Model file for the job. Use its own axes, mm. A direction names the side the tool comes from. Coordinates: 2 decimals unless noted, no trailing zeros. Write each loop counter-clockwise with the first axis right and the second up, starting at its lowest first coordinate (ties: lowest second). Pieces come first, ordered by that corner, then holes. Notation, with made-up numbers: M 28.25,75 L 80.25,75 A32 ccw 80.25,113 Z; hole C 29.25,84.5 d6. An arc over 180 degrees is marked long. Put each result on its own line as item: value. Start each with the question number.
Q1. Drop flat-ended pins along their axis: pin 1 (2.5 mm diameter, centred on x = 0.5, z = 25.5, fed in from +Y); pin 2 (1 mm diameter, centred on y = 1, z = 28.5, fed in from -X); pin 3 (1.5 mm diameter, centred on x = -1.5, z = 19.5, fed in from +Y). Give the stop position or say it passes through.
Q2. Cut at B-B (z = 13.5). Write the cut outline in (x, y).
Q3. Which spindle directions (+Z, -Z, +X, -X, +Y, -Y) get a long thin tool onto all of the face, cutting with end or side? Do faces 4 (the flat face through (0, 2, 8)), 5 (the cylindrical face through (-2.8, 0.1, 34.6)), 6 (the cylindrical face through (-3, 0.1, 35.2)). Say none if no direction does.
Q4. Pull direction Z, two halves, no side cores. Call faces 1 (the cylindrical face through (-0.65, -2.93, 17.77)), 2 (the flat face through (0, 1.5, 10)), 3 (the flat face through (0, 0, 36)): pulls with the +Z half, pulls with the -Z half, needs draft (parallel to the pull), parting line crosses it, or undercut.
Q5. Drill centre lines: line 1 along Z through (x, y) = (-1.7, 1.65); line 2 along X through (y, z) = (0.15, 4); line 3 along Y through (x, z) = (2.2, 2.5). Where is each one in solid material? Low to high.
Q6. Cut at C-C (y = 2). Give the number of separate pieces and of enclosed holes in the cut face, then the cut area to 3 significant figures.
```python
from build123d import *

# Parameters (mm, degrees)
SZKIC1_R                    = 3
DODANIE_WYCI_GNI_CIE1_DEPTH = 36
SFAZOWANIE1_SIZE            = 0.5
WYTNIJ_WYCI_GNI_CIE1_START  = -1.7
SZKIC2_R                    = 3
SZKIC2_R_2                  = 2.8
WYTNIJ_WYCI_GNI_CIE1_DEPTH  = 0.7
WYTNIJ_WYCI_GNI_CIE2_START  = -1
SZKIC3_R                    = 3
SZKIC3_R_2                  = 2.8
WYTNIJ_WYCI_GNI_CIE2_DEPTH  = 0.7
WYTNIJ_WYCI_GNI_CIE3_START  = -13
WYTNIJ_WYCI_GNI_CIE3_DEPTH  = 5
WYTNIJ_WYCI_GNI_CIE4_START  = -28
WYTNIJ_WYCI_GNI_CIE4_DEPTH  = 5


with BuildPart() as part:
    # Szkic1 → Dodanie-wyci_gni_cie1 (new body)
    with BuildSketch(Plane.XY):
        Circle(SZKIC1_R)
    extrude(amount=DODANIE_WYCI_GNI_CIE1_DEPTH)

    # Sfazowanie1
    sfazowanie1_edges = [part.edges().sort_by_distance(p)[0] for p in [
        (-3, 0, 0),
        (-3, 0, 36),
    ]]
    chamfer(sfazowanie1_edges, length=SFAZOWANIE1_SIZE)

    # Szkic2 → Wytnij-wyci_gni_cie1 (cut)
    with BuildSketch(Plane.XY.offset(36).offset(WYTNIJ_WYCI_GNI_CIE1_START)):
        Circle(SZKIC2_R)
        Circle(SZKIC2_R_2, mode=Mode.SUBTRACT)
    extrude(amount=WYTNIJ_WYCI_GNI_CIE1_DEPTH, mode=Mode.SUBTRACT)

    # Szkic3 → Wytnij-wyci_gni_cie2 (cut)
    with BuildSketch(Plane(origin=(0, 0, 0), x_dir=(-1, 0, 0), z_dir=(0, 0, -1)).offset(WYTNIJ_WYCI_GNI_CIE2_START)):
        Circle(SZKIC3_R)
        with Locations(Location((0, 0, 0), (0, 0, 180))):
            Circle(SZKIC3_R_2, mode=Mode.SUBTRACT)
    extrude(amount=-WYTNIJ_WYCI_GNI_CIE2_DEPTH, mode=Mode.SUBTRACT)

    # Szkic4 → Wytnij-wyci_gni_cie3 (cut)
    with BuildSketch(Plane.XY.offset(36).offset(WYTNIJ_WYCI_GNI_CIE3_START)):
        with BuildLine():
            Line((-2.598076211, 1.5), (2.598076211, 1.5))
            ThreePointArc((2.598076211, 1.5), (0, 3), (-2.598076211, 1.5))
        make_face()
    extrude(amount=WYTNIJ_WYCI_GNI_CIE3_DEPTH, mode=Mode.SUBTRACT)

    # Szkic4_2 → Wytnij-wyci_gni_cie4 (cut)
    with BuildSketch(Plane.XY.offset(36).offset(WYTNIJ_WYCI_GNI_CIE4_START)):
        with BuildLine():
            Line((-2.598076211, 1.5), (2.598076211, 1.5))
            ThreePointArc((2.598076211, 1.5), (0, 3), (-2.598076211, 1.5))
        make_face()
    extrude(amount=WYTNIJ_WYCI_GNI_CIE4_DEPTH, mode=Mode.SUBTRACT)


solid = part.part
```
Computed values:
1. pin 1: y = 1.5
1. pin 2: x = -2.96
1. pin 3: y = 2.9
2. outline: C 0,0 d6
3. face 4: +X, -X, +Y
3. face 5: none
3. face 6: +Z, -Z
4. face 1: needs draft
4. face 2: undercut
4. face 3: pulls with the +Z half
5. line 1: 0 to 8, 13 to 23, 28 to 36
5. line 2: -3 to 3
5. line 3: -2.04 to 2.04
6. separate pieces: 3
6. enclosed holes: 0
6. area: 115 mm2
